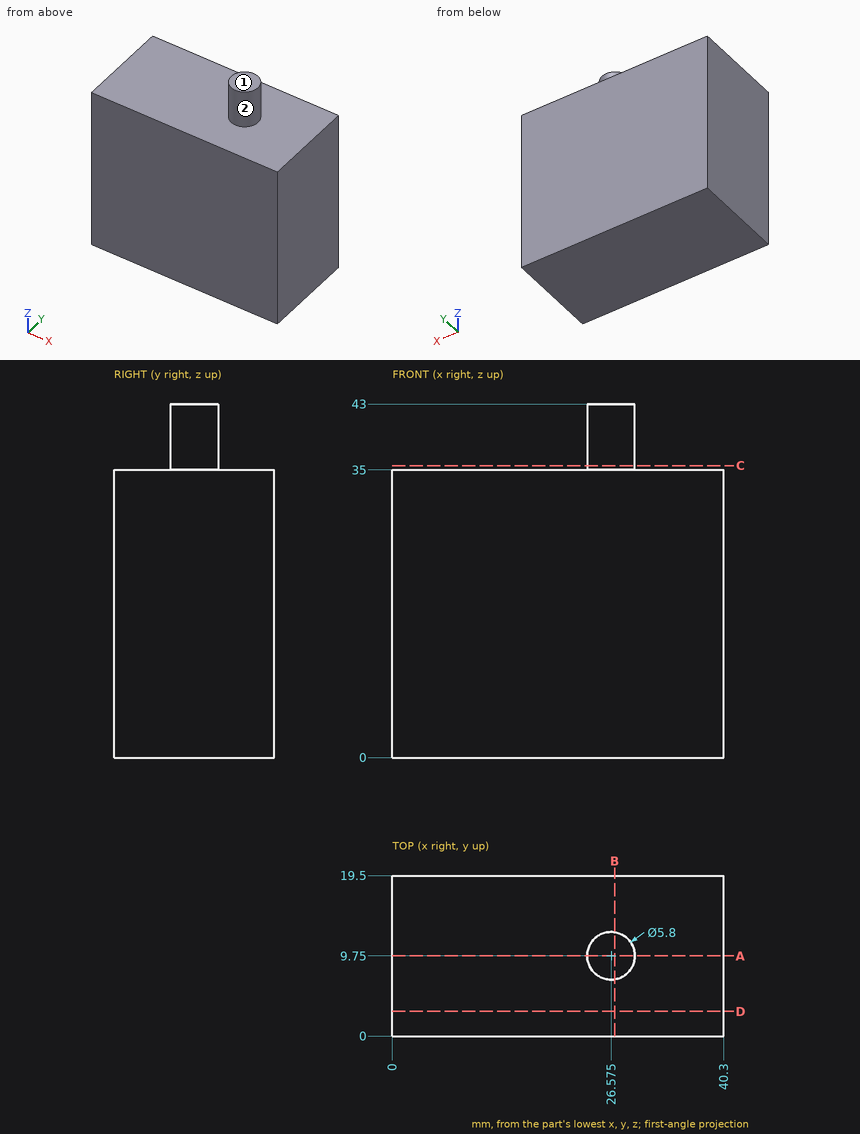
Input: dimensioned drawing with shaded views. Units: mm. Origin: part minimum x, y, z. A direction names the side the tool comes from. Coordinates: 2 decimals unless noted, no trailing zeros. Loops run counter-clockwise (first coordinate to the right, second up) from the corner with the lowest first, then second, coordinate; pieces in that order, holes last.
Q1. Line query: line 1 along Z through (x, y) = (32.5, 2.5); line 2 along X through (y, z) = (9.5, 40.5). Output: solid intervals per line, ascending.
Results are:
line 1: z = 0 to 35
line 2: x = 23.69 to 29.46
Q2. Contact query for a flat-ended pin moving along its axis: pin 1 (6 mm diameter, centred on x = 16.5, z = 26, fed in from -Y). Output: stop coordinate, or through.
Results are:
pin 1: stops at y = 0
Q3. Set-up query: the marked faces 1 and 2. Return all of +Z, -Z, +X, -X, +Y, -Y with unobstructed straight access to the full face (end or side cutting, diameter ignored); none if empty.
Results are:
face 1: +Z, +X, -X, +Y, -Y
face 2: +Z
Q4. Section A-A, the plane y = 9.75. Return the cut outline in (x, z) (3 decimals).
Results are:
outline: (0, 0) - (40.3, 0) - (40.3, 35) - (29.475, 35) - (29.475, 43) - (23.675, 43) - (23.675, 35) - (0, 35) - close
Q5. Section D-D, the plane y = 3. Return the cut outline in (x, z).
Results are:
outline: (0, 0) - (40.3, 0) - (40.3, 35) - (0, 35) - close
Q6. Section C-C, the plane z = 35.5. Return the cut outline in (x, y) (3 decimals), and give its area (3 significant figures).
Results are:
outline: circle Ø5.8 at (26.575, 9.75)
area: 26.4 mm2
Q7. Section B-B, the plane x = 27. Return the cut outline in (y, z), and give its area (3 significant figures).
Results are:
outline: (0, 0) - (19.5, 0) - (19.5, 35) - (12.62, 35) - (12.62, 43) - (6.88, 43) - (6.88, 35) - (0, 35) - close
area: 728 mm2
